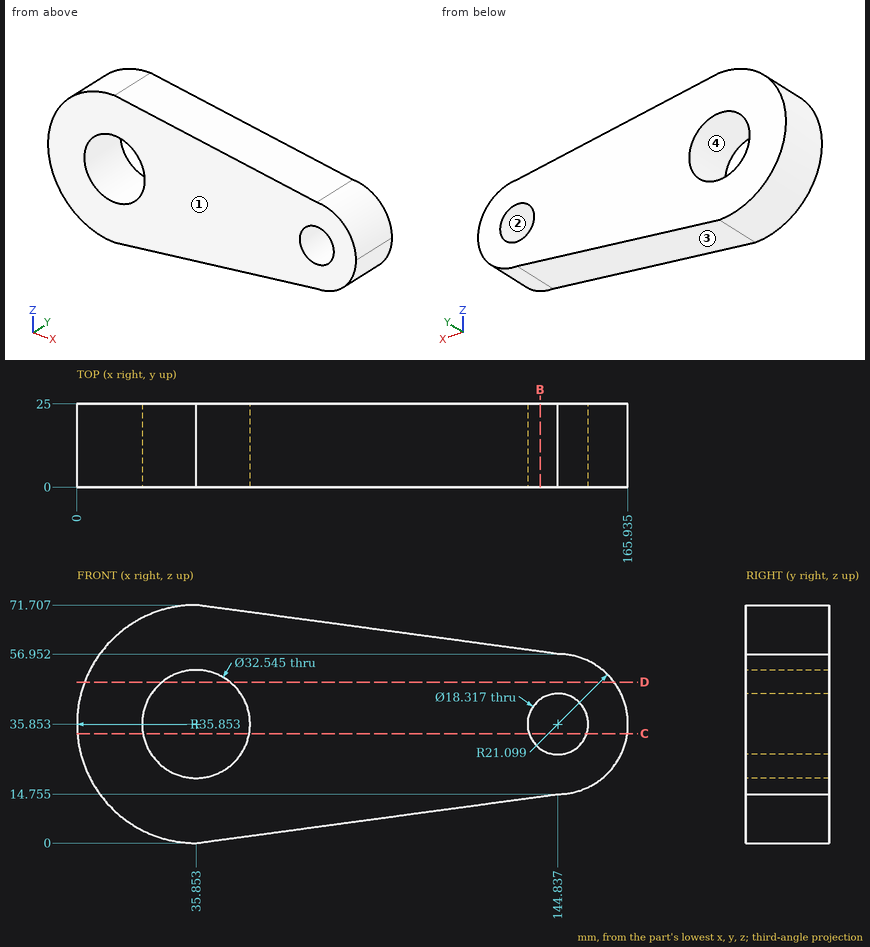
Here's the drawing with two shaded views (mm, measured from the low corner). I have some questions. Round coordinates to 2 decimals unless told otherwise and drop trailing zeros. Loops run counter-clockwise (first coordinate to the right, second up) from the corner with the lowest first, then second, coordinate; pieces in that order, holes last.
1. Suppose I cut it at B-B, the plane x = 139.5. Please give me the cut outline in (y, z) (1 decimal).
Answers:
outline: (0, 14) - (25, 14) - (25, 28.4) - (0, 28.4) - close; (0, 43.3) - (25, 43.3) - (25, 57.7) - (0, 57.7) - close
2. Suppose I cut it at D-D, the plane z = 48.5. Please give me the cut outline in (x, y) (1 decimal), and give its area (3 significant figures).
Answers:
outline: (2.3, 0) - (25.6, 0) - (25.6, 25) - (2.3, 25) - close; (46.1, 0) - (161.7, 0) - (161.7, 25) - (46.1, 25) - close
area: 3,470 mm2
3. Suppose I cut it at C-C, the plane z = 33. Please give me the cut outline in (x, y), and give its area (3 significant figures).
Answers:
outline: (0.11, 0) - (19.83, 0) - (19.83, 25) - (0.11, 25) - close; (51.87, 0) - (136.13, 0) - (136.13, 25) - (51.87, 25) - close; (153.54, 0) - (165.74, 0) - (165.74, 25) - (153.54, 25) - close
area: 2,900 mm2
4. If I drill on probe 1 along X at (y, z) = (3, 35) (1 decimal); probe 2 along X at (y, z) = (13, 39.5) (1 decimal); probe 3 along Z at (x, y) = (35.5, 11.5) (1 decimal), over which ranges is the centre line in solid material (lowest first)?
Answers:
probe 1: x = 0 to 19.6, 52.1 to 135.7, 154 to 165.9
probe 2: x = 0.2 to 20, 51.7 to 136.4, 153.2 to 165.6
probe 3: z = 0 to 19.6, 52.1 to 71.7
5. Will these pins go through, and if not, where does the flat tip stop? pin 1 (3 mm diameter, centred on y = 7, z = 18, fed in from -X); pin 2 (12 mm diameter, centred on x = 53, y = 3.5, fed in from +Z); pin 3 (2 mm diameter, centred on x = 88, y = 12, fed in from +Z).
Answers:
pin 1: stops at x = 3.95
pin 2: stops at z = 70.2
pin 3: stops at z = 64.78
6. Thinking about a two-plate mould opening in X: for the marked faces 1, 2, 3 and 4, which applies, released by +X, released by -X, zero draft, split by the parting line, or undercut?
Answers:
face 1: zero draft
face 2: undercut
face 3: released by +X
face 4: undercut
